Here's how the part is built. I have some questions about the finished solid (model axes, mm). Face numbers are marked on the shaded views. A direction names the side the tool comes from. Round coordinates to 2 decimals unless told otherwise and drop trailing zeros. Write each loop counter-clockwise with the first axis right and the second up, starting at its lowest first coordinate (ties: lowest second). Pieces come first, ordered by that corner, then holes. Notation, with made-up numbers: (56.25, -38.5) - (113.25, -38.5) arc R11 cw to (113.25, -24.5) - close; hole circle Ø9 at (50.5, 37.5). An arc over 180 degrees is marked (long way). One line per item, written item: value. Start each with the question number.
Item 1: For the marked faces 1 and 2, which set-ups out of +Z, -Z, +X, -X, +Y, -Y let a thin tool reach every point of the face, with its end or its side?
Item 2: Imagine slicing it at B-B, the plane x = -144.5. Please give me the cut outline in (y, z).
Item 3: Imagine slicing it at A-A, the plane x = -129.75. Please give me the cut outline in (y, z), then the cut area to 3 significant figures.
Item 4: Imagine slicing it at C-C, the plane z = -1.4. Count the separate pieces of the cut face and the enclosed holes in it, then the cut area to 3 significant figures.
Item 5: If I drill on line 1 (Z direction, x = -137.75, y = 13.5); line 2 (X direction, y = 22.5, z = -1.4); line 3 (X direction, y = 20.5, z = -2.15), over which ranges is the centre line in solid material (lowest first)?
Item 6: Thinking about a two-plate mould opening in Y: for the marked faces 3, 4 and 5, which applies, released by +Y, released by -Y, zero draft, split by the parting line, or undercut?
Item 7: For P1, Ø5, axis at x = -138.5, y = 1, coming from the -Z side; P2, Ø1.5, axis at y = 8, z = -1, coming from the +X side; P3, Ø1.5, axis at x = -131.5, z = -2.5, coming from the +Y side, each with a flat end and sliding along its axis, tell me the tip position at first contact or that it passes through.
Autodesk Inventor part; units mm, degrees
ref_plane "YZ Plane" through (0, 0, 0) normal (1, 0, 0) x (0, 1, 0)
ref_plane "XZ Plane" through (0, 0, 0) normal (0, 1, 0) x (-1, 0, 0)
ref_plane "XY Plane" through (0, 0, 0) normal (0, 0, 1) x (1, 0, 0)
sketch "スケッチ1" plane through (0, 0, 0) normal (0, 0, 1) x (1, 0, 0)
  circle A0 centre (-84.1159, 33.5789) radius 1.5
  circle A1 centre (-105.2485, 37.922) radius 1.5
  circle A2 centre (-132.6852, 21.2646) radius 1.5
  circle A3 centre (-77.8119, 54.5794) radius 1.5
  circle A4 centre (-112.1063, 12.5661) radius 1.5
  circle A5 centre (-60.4494, 64.5064) radius 1.5
  circle A6 centre (-64.4423, 49.0046) radius 1.5
  circle A7 centre (-44.4492, 64.0137) radius 1.5
  line L0 (-44.233, 71.0354) -> (-60.2332, 71.5281)
  arc A8 (-60.2332, 71.5281) -> (-64.0951, 70.5113) centre (-60.4494, 64.5064) ccw
  line L1 (-64.0951, 70.5113) -> (-153.1544, 16.4415)
  arc A9 (-153.1544, 16.4415) -> (-154.1888, 0.0236) centre (-147.9517, 7.8722) ccw
  line L2 (-154.1888, 0.0236) -> (-141.4408, -10.1069)
  arc A10 (-141.4408, -10.1069) -> (-131.6607, -10.2415) centre (-136.4636, -3.8437) ccw
  arc A11 (-40.2316, 58.3956) -> (-44.233, 71.0354) centre (-44.4492, 64.0137) ccw
  circle A12 centre (-147.9517, 7.8722) radius 1.5
  circle A13 centre (-136.4636, -3.8437) radius 1.5
  circle A14 centre (-132.6852, 21.2646) radius 1.5
  circle A15 centre (-132.6852, 21.2646) radius 4.5
  circle A16 centre (-147.9517, 7.8722) radius 4.5
  circle A17 centre (-136.4636, -3.8437) radius 1.5
  circle A18 centre (-136.4636, -3.8437) radius 4.5
  line L3 (-151.1648, 4.7216) -> (-139.6766, -6.9943)
  line L4 (-132.0137, -4.5133) -> (-128.2279, 20.6438)
  line L5 (-135.6527, 24.6475) -> (-150.9193, 11.255)
  circle A19 centre (-112.1063, 12.5661) radius 4.5
  point P0 (0, 0)
  point P1 (0, 0)
  point P2 (-128.2353, 20.595)
  dimension "d0" = 9
  dimension "d1" = 9
  dimension "d2" = 9
  dimension "d5" = 9
extrude "押し出し1" add sketch "スケッチ1" against normal blind 3 contours A15 L4 A18 L3 A16 L5 | A16 | A18
sketch "スケッチ2" plane through (0, 0, 0) normal (0, 0, 1) x (1, 0, 0)
  circle A0 centre (-142.0156, -13.6386) radius 1.5
  line L0 (-193.8461, -47.1997) -> (-168.4977, -27.8921)
  arc A1 (-162.0848, -31.6046) -> (-168.4977, -27.8921) centre (-166.0653, -31.0855) ccw
  line L1 (-162.0848, -31.6046) -> (-161.5284, -29.669)
  arc A2 (-161.365, -29.2693) -> (-161.5284, -29.669) centre (-159.6062, -30.2215) ccw
  line L2 (-161.365, -29.2693) -> (-154.7883, -17.1215)
  arc A3 (-151.2707, -19.0259) -> (-154.7883, -17.1215) centre (-153.0295, -18.0737) ccw
  line L3 (-151.2707, -19.0259) -> (-154.509, -25.0074)
  arc A4 (-154.509, -25.0074) -> (-153.0293, -26.2832) centre (-153.6296, -25.4835) ccw
  line L4 (-153.0293, -26.2832) -> (-128.1569, -7.6112)
  arc A5 (-128.1569, -7.6112) -> (-126.988, -5.6349) centre (-129.958, -5.212) ccw
  line L5 (-126.988, -5.6349) -> (-123.9066, 16.0052)
  arc A6 (-123.9066, 16.0052) -> (-127.0915, 19.4204) centre (-126.8767, 16.4281) ccw
  line L6 (-127.0915, 19.4204) -> (-130.5344, 19.1732)
  arc A7 (-134.5152, 18.8875) -> (-130.5344, 19.1732) centre (-132.6852, 21.2646) ccw
  line L7 (-134.5152, 18.8875) -> (-148.6695, 17.8715)
  arc A8 (-148.6695, 17.8715) -> (-157.1727, 11.806) centre (-147.9517, 7.8722) ccw
  line L8 (-157.1727, 11.806) -> (-166.1369, -9.2063)
  line L9 (-166.1369, -9.2063) -> (-193.8461, -47.1997)
  circle A9 centre (-126.8767, 16.4281) radius 1.5
  circle A10 centre (-158.5928, -9.2025) radius 1.5
  arc A11 (-128.5265, 10.8915) -> (-134.9494, 9.8931) centre (-131.7379, 10.3923) ccw
  arc A12 (-133.9759, -5.9529) -> (-128.5265, 10.8915) centre (-147.9517, 7.8722) ccw
  arc A13 (-138.597, -1.3817) -> (-133.9759, -5.9529) centre (-136.2864, -3.6673) ccw
  arc A14 (-138.597, -1.3817) -> (-134.9494, 9.8931) centre (-147.9517, 7.8722) ccw
  circle A15 centre (-147.9517, 7.8722) radius 4.025
  arc A16 (-150.9193, 11.255) -> (-151.1648, 4.7216) centre (-147.9517, 7.8722) ccw
  line L10 (-151.1648, 4.7216) -> (-139.6766, -6.9943)
  arc A17 (-139.6766, -6.9943) -> (-132.0137, -4.5133) centre (-136.4636, -3.8437) ccw
  line L11 (-132.0137, -4.5133) -> (-128.2353, 20.595)
  arc A18 (-128.2353, 20.595) -> (-135.6527, 24.6475) centre (-132.6852, 21.2646) ccw
  line L12 (-135.6527, 24.6475) -> (-150.9193, 11.255)
  circle A19 centre (-132.6852, 21.2646) radius 1.5
  circle A20 centre (-147.9517, 7.8722) radius 1.5
  circle A21 centre (-136.4636, -3.8437) radius 1.5
  circle A22 centre (-126.8767, 16.4281) radius 3.25
  point P0 (0, 0)
  point P1 (0, 0)
  dimension "d6" = 6.5
extrude "押し出し2" cut sketch "スケッチ2" against normal blind 10 contours A22 L5 A6 L6 | L6 A6 L5 A22 L11 | L11 A22 | A9
sketch "スケッチ3" plane through (0, 0, -3) normal (0, 0, -1) x (-1, 0, 0)
  arc A0 (129.2038, 14.1593) -> (128.433, 19.2812) centre (126.8767, 16.4281) ccw
  line L0 (129.2038, 14.1593) -> (132.0137, -4.5133)
  arc A1 (132.0137, -4.5133) -> (139.6766, -6.9943) centre (136.4636, -3.8437) ccw
  line L1 (139.6766, -6.9943) -> (151.1648, 4.7216)
  arc A2 (151.1648, 4.7216) -> (150.9193, 11.255) centre (147.9517, 7.8722) ccw
  line L2 (150.9193, 11.255) -> (135.6527, 24.6475)
  arc A3 (135.6527, 24.6475) -> (128.2353, 20.595) centre (132.6852, 21.2646) ccw
  line L3 (128.2353, 20.595) -> (128.433, 19.2812)
  circle A4 centre (132.6852, 21.2646) radius 1.5
  circle A5 centre (147.9517, 7.8722) radius 1.5
  circle A6 centre (136.4636, -3.8437) radius 1.5
  line L4 (149.0228, 6.822) -> (137.5346, -4.8939)
  arc A7 (134.9803, -4.0669) -> (137.5346, -4.8939) centre (136.4636, -3.8437) ccw
  line L5 (134.9803, -4.0669) -> (132.3502, 13.4109)
  arc A8 (132.3502, 13.4109) -> (131.2198, 20.9225) centre (126.8767, 16.4281) ccw
  line L6 (131.2198, 20.9225) -> (131.2019, 21.0414)
  arc A9 (133.6744, 22.3923) -> (131.2019, 21.0414) centre (132.6852, 21.2646) ccw
  line L7 (133.6744, 22.3923) -> (148.9409, 8.9998)
  arc A10 (149.0228, 6.822) -> (148.9409, 8.9998) centre (147.9517, 7.8722) ccw
  circle A11 centre (132.6852, 21.2646) radius 1.5
  circle A12 centre (132.6852, 21.2646) radius 4.5
  circle A13 centre (147.9517, 7.8722) radius 4.5
  circle A14 centre (136.4636, -3.8437) radius 1.5
  circle A15 centre (136.4636, -3.8437) radius 4.5
  point P0 (0, 0)
  point P1 (134.349, 0.1285)
  point P2 (140.505, -1.8646)
  point P3 (146.0523, 3.7927)
  point P4 (145.7516, 11.7976)
  point P5 (136.8637, 19.5944)
  point P6 (133.1164, 16.7854)
  dimension "d9" = 3
extrude "押し出し3" cut sketch "スケッチ3" against normal blind 2.5 contours A12 L7 A13 L4 A15 L5 A8
sketch "スケッチ4" plane through (0, 0, -3) normal (0, 0, -1) x (-1, 0, 0)
  line L0 (140.505, -1.8646) -> (146.0523, 3.7927)
  arc A0 (145.7516, 11.7976) -> (146.0523, 3.7927) centre (147.9517, 7.8722) ccw
  line L1 (145.7516, 11.7976) -> (136.8637, 19.5944)
  arc A1 (133.1164, 16.7854) -> (136.8637, 19.5944) centre (132.6852, 21.2646) ccw
  arc A2 (132.3502, 13.4109) -> (133.1164, 16.7854) centre (126.8767, 16.4281) ccw
  line L2 (132.3502, 13.4109) -> (134.349, 0.1285)
  arc A3 (140.505, -1.8646) -> (134.349, 0.1285) centre (136.4636, -3.8437) ccw
  circle A4 centre (136.4636, -3.8437) radius 1.5
  circle A5 centre (147.9517, 7.8722) radius 1.5
  circle A6 centre (132.6852, 21.2646) radius 1.5
  line L3 (151.1648, 4.7216) -> (139.6766, -6.9943)
  arc A7 (132.0137, -4.5133) -> (139.6766, -6.9943) centre (136.4636, -3.8437) ccw
  line L4 (132.0137, -4.5133) -> (129.2038, 14.1593)
  arc A8 (129.2038, 14.1593) -> (128.433, 19.2812) centre (126.8767, 16.4281) ccw
  line L5 (128.433, 19.2812) -> (128.2353, 20.595)
  arc A9 (135.6527, 24.6475) -> (128.2353, 20.595) centre (132.6852, 21.2646) ccw
  line L6 (135.6527, 24.6475) -> (150.9193, 11.255)
  arc A10 (151.1648, 4.7216) -> (150.9193, 11.255) centre (147.9517, 7.8722) ccw
  line L7 (147.9517, 7.8722) -> (132.6852, 21.2646) construction
  line L8 (148.9409, 8.9998) -> (133.6744, 22.3923)
  line L9 (131.696, 20.137) -> (146.9626, 6.7446)
  arc A11 (146.9626, 6.7446) -> (148.9409, 8.9998) centre (147.9517, 7.8722) ccw
  arc A12 (133.6744, 22.3923) -> (131.696, 20.137) centre (132.6852, 21.2646) ccw
  circle A13 centre (132.6852, 21.2646) radius 4.5
  circle A14 centre (147.9517, 7.8722) radius 4.5
  point P0 (0, 0)
  point P1 (140.3185, 14.5684)
  point P2 (145.7516, 11.7976)
  point P3 (135.6527, 24.6475)
  point P4 (134.8854, 17.3392)
  point P5 (143.7732, 9.5424)
  dimension "d12" = 3
extrude "押し出し4" cut sketch "スケッチ4" against normal blind 10 contours L1 A13 L6 A14
extrude "押し出し5" add sketch "スケッチ4" against normal blind 3 contours L9 A1 L1 A0
sketch "スケッチ5" plane through (0, 0, -3) normal (0, 0, -1) x (-1, 0, 0)
  point P0 (0, 0)
fillet "フィレット1" radius 1 7 edges at (-134.8854, 17.3392, -1.75) (-133.1164, 16.7854, -1.75) (-132.3502, 13.4109, -1.75) (-143.7732, 9.5424, -1.75) (-146.0523, 3.7927, -1.75) (-140.505, -1.8646, -1.75) (-134.349, 0.1285, -1.75)
fillet "フィレット2" radius 1 2 edges at (-136.8637, 19.5944, -1.5) (-145.7516, 11.7976, -1.5)
properties part number "アーム ツインアーム先端押さえ" material "ポリカーボネート、クリア"
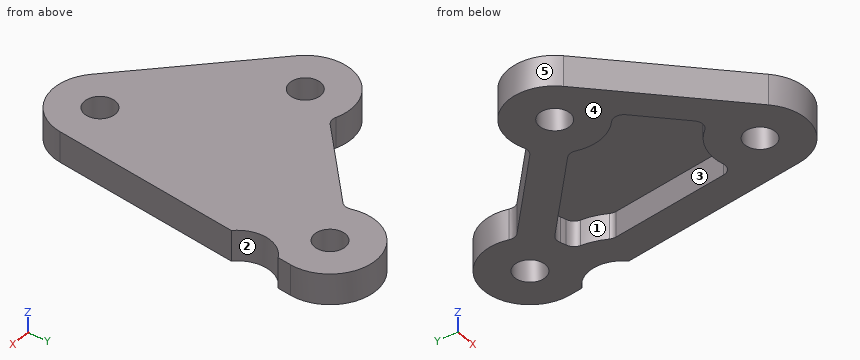
Values follow:
1. face 1: -Z
1. face 2: +Z, -Z, +X
2. outline: (-2.08, -3) - (2.21, -3) - (2.21, -0.5) - (4.99, -0.5) - (4.99, -3) - (12.9, -3) - (12.9, 0) - (-2.08, 0) - close
3. outline: (10.53, -3) - (14.91, -3) - (14.91, 0) - (10.53, 0) - close; (17.95, -3) - (24.68, -3) - (24.68, 0) - (17.95, 0) - close
3. area: 33.3 mm^2
4. separate pieces: 1
4. enclosed holes: 4
4. area: 292 mm^2
5. line 1: z = -0.5 to 0
5. line 2: x = -137.01 to -133.54, -131.83 to -128.36
5. line 3: x = -137.12 to -133.98, -131.39 to -128.25
6. face 3: undercut
6. face 4: zero draft
6. face 5: split by the parting line
7. P1: stops at z = -3
7. P2: stops at x = -130.02
7. P3: stops at y = 25.74
